Geometry check sheet. Reference: drawing and pictorial views, mm from the part's lowest x, y, z. A direction names the side the tool comes from. Round coordinates to 2 decimals unless told otherwise and drop trailing zeros. Order: outer loops, then holes, each group sorted by start corner. A loop starts at its lowest first (then second) coordinate and runs counter-clockwise, first axis right, second up.
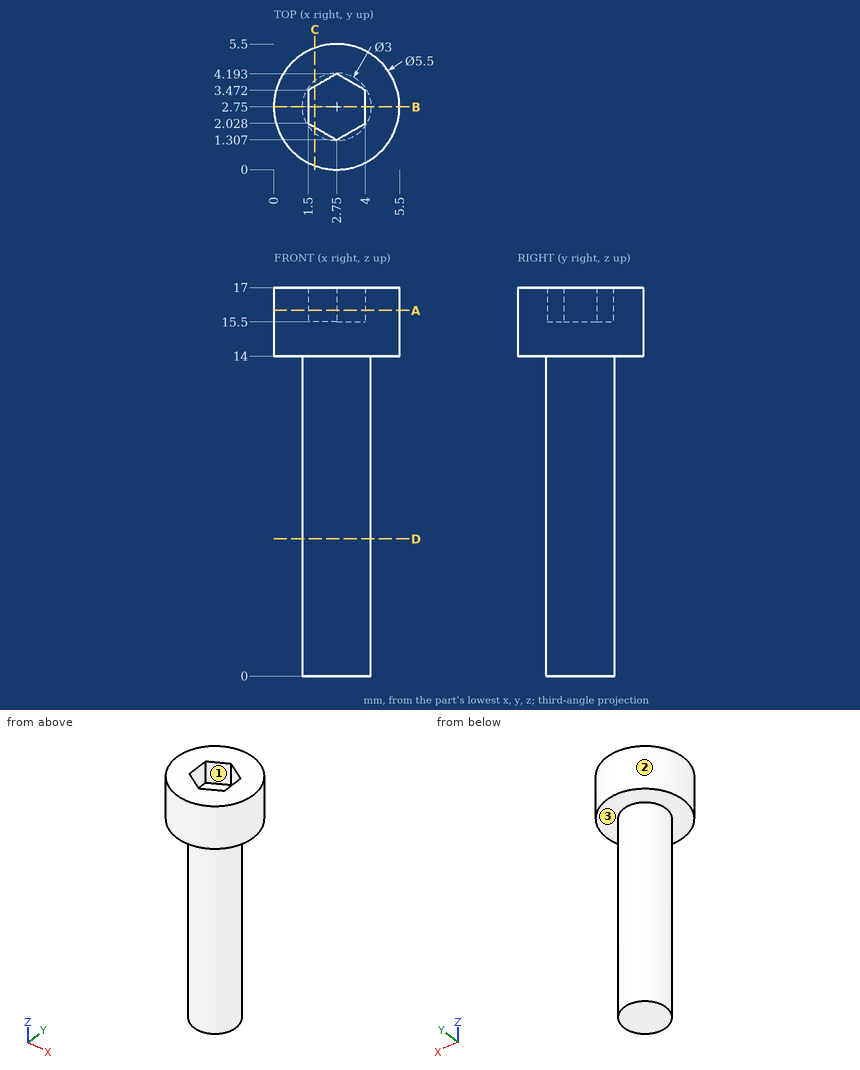
1) Scan lines: probe 1 along Z at (x, y) = (2.55, 3.65); probe 2 along Z at (x, y) = (1.1, 4); probe 3 along X at (y, z) = (2.65, 7.5). Record each from-to range of solid material in increasing order.
2) Sectioned sample at C-C on x = 1.8. Record the cut outline in (y, z) (1 decimal), then the cut area to 3 significant figures.
3) Sectioned sample at B-B on y = 2.75. Record the cut outline in (x, z).
4) Sectioned sample at D-D on z = 6. Record the cut outline in (x, y).
5) Sectioned sample at A-A on z = 16. Record the cut outline in (x, y).
6) Go/stop test with flat-tipped pins: pin 1 Ø1.2 at (x, y) = (2.5, 3) entering from +Z; pin 2 Ø2 at (y, z) = (2.5, 12.5) entering from +X; pin 3 Ø2 at (x, z) = (2.5, 11) entering from -Y. Record where each tip stops, or that it passes through.
7) Tool access check on the marked faces 1, 2 and 3. Record the directions out of +Z, -Z, +X, -X, +Y, -Y that give a thin tool (end or side, any length) a straight path to the whole face; none if there is none.
Returned:
1. probe 1: z = 0 to 15.5
1. probe 2: z = 14 to 17
1. probe 3: x = 1.25 to 4.25
2. outline: (0.2, 14) - (1.6, 14) - (1.6, 0) - (3.9, 0) - (3.9, 14) - (5.3, 14) - (5.3, 17) - (3.6, 17) - (3.6, 15.5) - (1.9, 15.5) - (1.9, 17) - (0.2, 17) - close
2. area: 45.3 mm2
3. outline: (0, 14) - (1.25, 14) - (1.25, 0) - (4.25, 0) - (4.25, 14) - (5.5, 14) - (5.5, 17) - (4, 17) - (4, 15.5) - (1.5, 15.5) - (1.5, 17) - (0, 17) - close
4. outline: circle Ø3 at (2.75, 2.75)
5. outline: circle Ø5.5 at (2.75, 2.75); hole (1.5, 2.03) - (2.75, 1.31) - (4, 2.03) - (4, 3.47) - (2.75, 4.19) - (1.5, 3.47) - close
6. pin 1: stops at z = 15.5
6. pin 2: stops at x = 4.25
6. pin 3: stops at y = 1.25
7. face 1: +Z
7. face 2: +Z, -Z
7. face 3: -Z
